Model file for the job. Use its own axes, mm. A direction names the side the tool comes from. Give positions to 0.01 mm unless a question says otherwise; leave off trailing zeros. Loops run counter-clockwise (first coordinate to the right, second up) from the corner with the lowest first, then second, coordinate; pieces in that order, holes last. Notation, with made-up numbers: M 71.5,79.25 L 94.5,79.25 A6 ccw 94.5,90.25 Z; hole C 70.5,40.5 d8. An arc over 180 degrees is marked long. Answer in a Markdown table with one row per item.
Autodesk Inventor part; units mm, degrees
ref_plane "Start Plane" through (0, 0, 0) normal (0, 0, 1) x (1, 0, 0)
ref_plane "End Plane" through (0, 0, 152.4) normal (0, 0, 1) x (1, 0, 0)
ref_plane "YZ Plane" through (0, 0, 0) normal (1, 0, 0) x (0, 1, 0)
ref_plane "Start Plane" through (0, 0, 0) normal (0, 0, 1) x (1, 0, 0)
ref_plane "End Plane" through (0, 0, 152.4) normal (0, 0, 1) x (1, 0, 0)
sketch "Sketch" plane through (0, 0, 0) normal (0, 0, 1) x (1, 0, 0)
  line L0 (-25.4, -12.7) -> (25.4, -12.7)
  line L1 (25.4, -12.7) -> (25.4, 12.7)
  line L2 (25.4, 12.7) -> (-25.4, 12.7)
  line L3 (-25.4, 12.7) -> (-25.4, -12.7)
  line L4 (-25.4, -12.7) -> (25.4, 12.7) construction
  line L5 (25.4, -12.7) -> (-25.4, 12.7) construction
  line L6 (-22.225, -9.525) -> (22.225, -9.525)
  line L7 (22.225, -9.525) -> (22.225, 9.525)
  line L8 (22.225, 9.525) -> (-22.225, 9.525)
  line L9 (-22.225, 9.525) -> (-22.225, -9.525)
  line L10 (-22.225, -9.525) -> (22.225, 9.525) construction
  line L11 (22.225, -9.525) -> (-22.225, 9.525) construction
  point P0 (0, 0)
  point P1 (0, 0)
  dimension "d0" = 50.8
  dimension "d1" = 25.4
  dimension "d2" = 3.175
  dimension "d3" = 3.175
extrude "Body" add sketch "Sketch" along normal up to surface (152.4 mm away) from surface at 0
sketch "Sketch4" plane through (0, 0, 0) normal (0, 0, 1) x (1, 0, 0)
  line L0 (0, 0) -> (10, 0)
ref_plane "Work Plane4" through (0, 0, 0) normal (0, -1, 0) x (1, 0, 0)
sketch "Sketch5" plane through (0, 0, 0) normal (0, -1, 0) x (1, 0, 0)
  line L0 (-2, 0) -> (12, 0)
  line L1 (-2, 152.4) -> (12, 152.4)
  dimension "d11" = 152.4
equation "\"G_OFFSET_START\" = 0"
equation "\"G_OFFSET_END\" = 0"
equation "\"d7\" = length + G_OFFSET_END"
equation "\"G_L\" = d11"
properties part number "2x1inTubing"
Q1. Mould opens along X. For faces 3 (the face through (22.225, 0, 75)), 4 (the face through (0, -12.7, 75)), 5 (the face through (-25.4, 0, 75)) say: released by +X, released by -X, zero draft, split by the parting line, or undercut.
Reported:
| item | result |
|---|---|
| face 3 | undercut |
| face 4 | zero draft |
| face 5 | released by -X |
Q2. Saw through at B-B (y = -3.25). Give the cut face in (x, z) (3 decimals).
Reported:
| item | result |
|---|---|
| outline | M -25.4,0 L -22.225,0 L -22.225,152.4 L -25.4,152.4 Z; M 22.225,0 L 25.4,0 L 25.4,152.4 L 22.225,152.4 Z |
Q3. Saw through at C-C (z = 131.5). Give the cut face in (x, y) (3 decimals).
Reported:
| item | result |
|---|---|
| outline | M -25.4,-12.7 L 25.4,-12.7 L 25.4,12.7 L -25.4,12.7 Z; hole M -22.225,-9.525 L 22.225,-9.525 L 22.225,9.525 L -22.225,9.525 Z |
Q4. Probe probe 1 along X at (y, z) = (8, 35) (3 decimals); probe 2 along Y at (x, z) = (-4.5, 44) (3 decimals). List the from-to ranges inside material, lowest first.
Reported:
| item | result |
|---|---|
| probe 1 | -25.4 to -22.225, 22.225 to 25.4 |
| probe 2 | -12.7 to -9.525, 9.525 to 12.7 |
Q5. 3-axis set-ups, long thin cutter, end or side, ignore diameter. For faces 1 (the face through (0, 9.525, 75)), 2 (the face through (0, 10, 152.4)): which of +Z, -Z, +X, -X, +Y, -Y reach the whole face in a straight line?
Reported:
| item | result |
|---|---|
| face 1 | +Z, -Z |
| face 2 | +Z, +X, -X, +Y, -Y |
Q6. Saw through at A-A (x = 0). Give the cut face in (y, z) (3 decimals).
Reported:
| item | result |
|---|---|
| outline | M -12.7,0 L -9.525,0 L -9.525,152.4 L -12.7,152.4 Z; M 9.525,0 L 12.7,0 L 12.7,152.4 L 9.525,152.4 Z |
